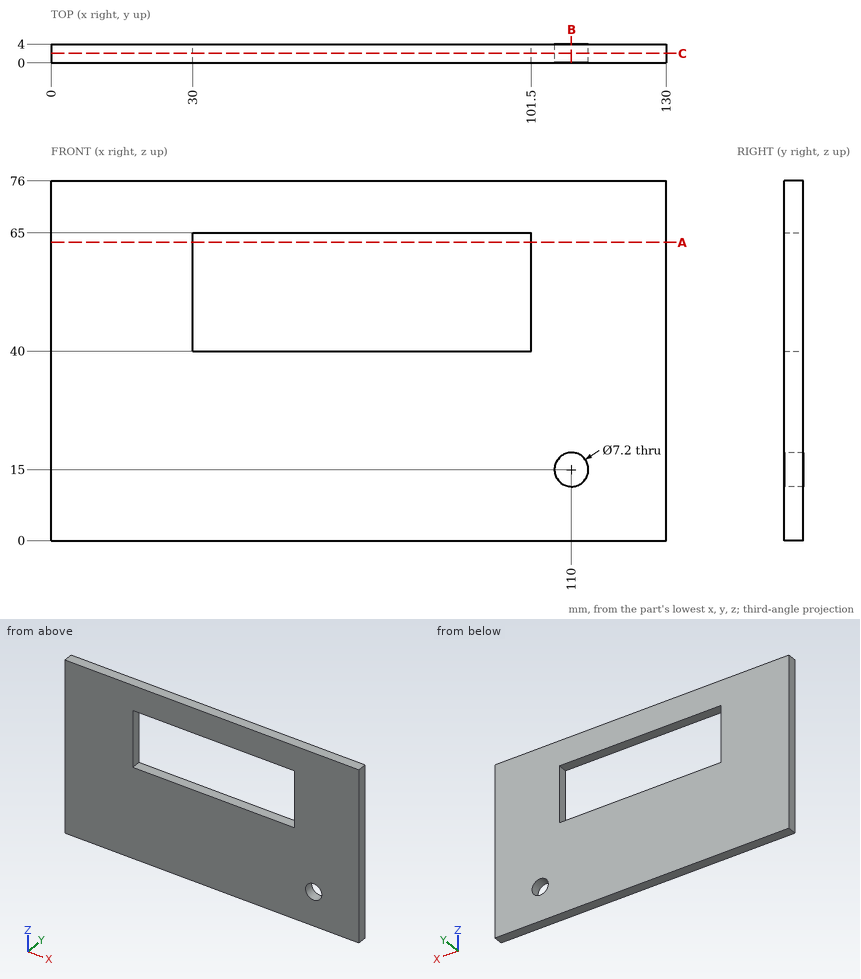
Input: dimensioned drawing with shaded views. Units: mm. Origin: part minimum x, y, z. Give positions to 0.01 mm unless a question says otherwise; leave off trailing zeros. Order: outer loops, then holes, each group sorted by start corner. A loop starts at its lowest first (then second) coordinate and runs counter-clockwise, first axis right, second up. Notation, with made-up numbers: (35.25, 86) -> (69.25, 86) arc R9 ccw to (69.25, 91) -> close; hole circle Ø7 at (32, 88). An arc over 180 degrees is marked (long way). Answer as a JSON object with one key per item and string values.
Q1. Section A-A (z = 63). Output: boundary loops of the cut face in (x, y).
Entries:
{"outline": "(0, 0) -> (30, 0) -> (30, 4) -> (0, 4) -> close; (101.5, 0) -> (130, 0) -> (130, 4) -> (101.5, 4) -> close"}
Q2. Material intervals for probe 1 along Z at (x, y) = (43.5, 3.8); probe 2 along X at (y, z) = (2.4, 58.5); probe 3 along Z at (x, y) = (110, 2.75), sorted ascending.
Entries:
{"probe 1": "z = 0 to 40, 65 to 76", "probe 2": "x = 0 to 30, 101.5 to 130", "probe 3": "z = 0 to 11.4, 18.6 to 76"}
Q3. Section B-B (x = 110). Output: boundary loops of the cut face in (y, z).
Entries:
{"outline": "(0, 0) -> (4, 0) -> (4, 11.4) -> (0, 11.4) -> close; (0, 18.6) -> (4, 18.6) -> (4, 76) -> (0, 76) -> close"}
Q4. Section C-C (y = 2). Output: boundary loops of the cut face in (x, z), plus the area to 3 significant figures.
Entries:
{"outline": "(0, 0) -> (130, 0) -> (130, 76) -> (0, 76) -> close; hole (30, 40) -> (101.5, 40) -> (101.5, 65) -> (30, 65) -> close; hole circle Ø7.2 at (110, 15)", "area": "8,050 mm^2"}
